Build history of the part. All positions in model axes, mm. A direction names the side the tool comes from. Round coordinates to 2 decimals unless told otherwise and drop trailing zeros. Order: outer loops, then holes, each group sorted by start corner. A loop starts at its lowest first (then second) coordinate and runs counter-clockwise, first axis right, second up. Notation, with made-up numbers: M 39.25,52 L 83.25,52 A34 cw 83.25,83 Z; hole C -33,36 d9. An arc over 180 degrees is marked long. One line per item, written item: value. Start each with the question number.
Item 1: Band-saw the part on B-B, the plane x = 32. Write the cut outline in (y, z), then the cut area to 3 significant figures.
Item 2: Pin check, flat tips, straight feed: pin 1 (3 mm diameter, centred on x = 41, z = 111.5, fed in from +Y); pin 2 (2 mm diameter, centred on x = 19, z = 171, fed in from +Y); pin 3 (2 mm diameter, centred on y = -10.5, z = 130.5, fed in from -X); pin 4 (7 mm diameter, centred on x = 33.19, y = -10.77, fed in from +Z). Stop position of each tip, or through.
Item 3: Tool access for faces 5 (the flat face through (28.191, 10, 98)), 6 (the flat face through (33, 13, 105)), 7 (the flat face through (33, 7.231, 98)), 8 (the flat face through (38.191, 10, 98)), 9 (the flat face through (20.672, -10, 149)): list every direction of +Z, -Z, +X, -X, +Y, -Y with a clear straight run to the whole face (end or side of a thin tool).
Item 4: Band-saw the part on A-A, the plane y = 18. Write the cut outline in (x, z), then the cut area to 3 significant figures.
Item 5: Band-saw the part on D-D, the plane y = 0.5. Write the cut outline in (x, z).
Item 6: Two-plate mould, pull along Z, no slides. Class faces 1 (the flat face through (33, 2, 215)), 2 (the flat face through (25.24, -3.45, 149.3)), 3 (the flat face through (33, 10, 95)), 4 (the flat face through (33, 13, 115)): +Z half, -Z half, draft (parallel to the pull), parting line (faces both ways), or undercut.
Item 7: Probe L1, parallel to Z at x = 46, y = 9; L2, parallel to Y at x = 28, z = 205; L3, parallel to X at y = -2, z = 183. List the from-to ranges inside material, lowest first.
Item 8: Band-saw the part on C-C, the plane z = 189.5. Write the cut outline in (x, y), then the cut area to 3 significant figures.
Autodesk Inventor part; units mm, degrees
ref_plane "YZ Plane" through (0, 0, 0) normal (1, 0, 0) x (0, 1, 0)
ref_plane "XZ Plane" through (0, 0, 0) normal (0, 1, 0) x (-1, 0, 0)
ref_plane "XY Plane" through (0, 0, 0) normal (0, 0, 1) x (1, 0, 0)
sketch "Эскиз1" plane through (0, 0, 0) normal (0, 0, 1) x (1, 0, 0)
  arc A0 (47.2167, -13.0271) -> (19.1654, -13.0271) centre (33.1911, 1.2306) ccw
  line L0 (26.6911, 1.9729) -> (39.6911, 1.9729)
  line L1 (39.6911, 1.9729) -> (42.6385, -9.0271)
  line L2 (33.1911, 1.9729) -> (33.1911, -13.0271) construction
  line L3 (26.6911, 1.9729) -> (23.7436, -9.0271)
  line L4 (22.6718, -13.0271) -> (22.6718, -11.0271)
  line L5 (22.6718, -11.0271) -> (20.6718, -11.0271)
  line L6 (20.6718, -11.0271) -> (20.6718, -9.0271)
  line L7 (20.6718, -9.0271) -> (23.7436, -9.0271)
  line L8 (43.7103, -13.0271) -> (43.7103, -11.0271)
  line L9 (43.7103, -11.0271) -> (45.7103, -11.0271)
  line L10 (45.7103, -11.0271) -> (45.7103, -9.0271)
  line L11 (45.7103, -9.0271) -> (42.6385, -9.0271)
  line L12 (19.1654, -13.0271) -> (22.6718, -13.0271)
  line L13 (43.7103, -13.0271) -> (47.2167, -13.0271)
  point P0 (19.1654, -13.0271)
  dimension "d3" = 13
  dimension "d4" = 105
  dimension "d5" = 15
  dimension "d6" = 40
  dimension "d44" = 2
  dimension "d45" = 2
  dimension "d46" = 2
  dimension "d47" = 3.5064
extrude "Выдавливание1" add sketch "Эскиз1" along normal blind 200
ref_plane "РабПлоскость2" through (0, 0, 105) normal (0, 0, 1) x (1, 0, 0)
ref_plane "РабПлоскость1" through (0, 0, 100) normal (0, 0, 1) x (1, 0, 0)
sketch "Эскиз3" plane through (0, 0, 200) normal (0, 0, 1) x (1, 0, 0)
  arc A0 (47.2167, -13.0271) -> (19.1654, -13.0271) centre (33.1911, 1.2306) ccw
  circle A1 centre (33.1911, 1.2306) radius 20
  point P0 (0, 0)
  point P1 (19.1654, -13.0271)
extrude "Выдавливание3" add sketch "Эскиз3" along normal blind 15
sketch "Эскиз5" plane through (33.1911, 1.2306, 215) normal (0, 0, 1) x (1, 0, 0)
  circle A0 centre (0, -12) radius 6
  circle A1 centre (0, 0) radius 20 construction
  circle A2 centre (0, 0) radius 18 construction
  circle A3 centre (0, 0) radius 20 construction
  line L0 (0, -20) -> (0, 0)
  point P0 (-33.1911, -1.2306)
  dimension "d38" = 12
  dimension "d39" = 2
extrude "Выдавливание5" cut sketch "Эскиз5" against normal blind 15
sketch "Эскиз13" plane through (0, 0, 105) normal (0, 0, 1) x (1, 0, 0)
  circle A0 centre (33.1911, 1.2306) radius 20
  circle A1 centre (33.1911, 1.2306) radius 20
  line L0 (14.1123, 7.2306) -> (52.2699, 7.2306)
  point P0 (0, 0)
  dimension "d79" = 6
extrude "Выдавливание12" cut sketch "Эскиз13" along normal blind 10 contours L0 A0 picked at (30.9346, 14.3004)
sketch "Эскиз14" plane through (0, 0, 0) normal (0, 0, -1) x (-1, 0, 0)
  arc A0 (-14.1123, 7.2306) -> (-52.2699, 7.2306) centre (-33.1911, 1.2306) ccw
  circle A1 centre (-33.1911, 1.2306) radius 20
  point P0 (0, 0)
  point P1 (-52.2699, 7.2306)
extrude "Выдавливание13" cut sketch "Эскиз14" against normal up to surface (100 mm away)
sketch "Эскиз15" plane through (33.1911, 1.2306, 100) normal (0, 0, -1) x (-1, 0, 0)
  line L0 (-5, 11) -> (5, 11)
  line L1 (5, 11) -> (5, 6)
  line L2 (5, 6) -> (-5, 6)
  line L3 (-5, 6) -> (-5, 11)
  arc A0 (19.0788, 6) -> (-19.0788, 6) centre (0, 0) ccw
  line L4 (0, 0) -> (0, 22.3404)
  point P0 (33.1911, -1.2306)
  point P1 (0, 11)
  dimension "d84" = 10
  dimension "d85" = 5
  dimension "d86" = 6
extrude "Выдавливание14" add sketch "Эскиз15" along normal blind 5
properties part number "lamp2"
Output:
1. outline: M -18.73,200 L -16.65,200 L -16.65,215 L -18.73,215 Z; M -4.89,200 L 1.97,200 L 1.97,100 L 7.23,100 L 7.23,95 L 12.23,95 L 12.23,100 L 21.2,100 L 21.2,105 L 7.23,105 L 7.23,115 L 21.2,115 L 21.2,215 L -4.89,215 Z
1. area: 2,230 mm²
2. pin 1: stops at y = 7.23
2. pin 2: stops at y = 16.26
2. pin 3: stops at x = 16.31
2. pin 4: passes through
3. face 5: -Z, -X, +Y, -Y
3. face 6: +X, -X, +Y
3. face 7: -Z, +X, -X, -Y
3. face 8: -Z, +X, +Y, -Y
3. face 9: -Z
4. outline: M 22.29,100 L 44.09,100 L 44.09,105 L 22.29,105 Z; M 22.29,115 L 44.09,115 L 44.09,215 L 22.29,215 Z
4. area: 2,290 mm²
5. outline: M 13.2,100 L 26.3,100 L 26.3,200 L 40.09,200 L 40.09,100 L 53.18,100 L 53.18,215 L 13.2,215 Z
6. face 1: +Z half
6. face 2: draft
6. face 3: -Z half
6. face 4: undercut
7. L1: z = 100 to 105, 115 to 215
7. L2: y = -18.08 to -13.78, -7.76 to 20.55
7. L3: x = 13.45 to 25.63, 40.76 to 52.93
8. outline: M 19.17,-13.03 L 22.67,-13.03 L 22.67,-11.03 L 20.67,-11.03 L 20.67,-9.03 L 23.74,-9.03 L 26.69,1.97 L 39.69,1.97 L 42.64,-9.03 L 45.71,-9.03 L 45.71,-11.03 L 43.71,-11.03 L 43.71,-13.03 L 47.22,-13.03 A20 ccw long Z
8. area: 878 mm²
